```python
from build123d import *

# Parameters (mm, degrees)
F1_DEPTH = 21
F2_R     = 5
F3_R     = 2
F4_DEPTH = 25
F5_R     = 4.5
F6_DEPTH = 4
F7_R     = 3


with BuildPart() as f1:
    # F0 (on Front) → F1 (new body)
    with BuildSketch(Plane.XZ):
        Polygon((95.5, 17), (6.891753, 17), (0, 17), (0, 0), (95.5, 0), align=None)
    extrude(amount=F1_DEPTH)

    # F2
    f2_edges = [f1.edges().sort_by_distance(p)[0] for p in [
        (95.5, -10.5, 17),
    ]]
    fillet(f2_edges, radius=F2_R)

    # F3 (on face) → F4 (cut)
    with BuildSketch(Plane.XY.offset(17)):
        with BuildLine():
            ThreePointArc((41.5, -10.5), (39.5, -8.5), (37.5, -10.5))
            ThreePointArc((37.5, -10.5), (39.5, -12.5), (41.5, -10.5))
        make_face()
        with BuildLine():
            ThreePointArc((7.75, -10.5), (9.75, -12.5), (11.75, -10.5))
            Line((11.75, -10.5), (7.75, -10.5))
        make_face()
        with BuildLine():
            Line((7.75, -10.5), (11.75, -10.5))
            ThreePointArc((11.75, -10.5), (9.75, -8.5), (7.75, -10.5))
        make_face()
        with Locations((78.5, -10.5)):
            Circle(F3_R)
    extrude(amount=-F4_DEPTH, mode=Mode.SUBTRACT)

    # F5 (on face) → F6 (cut)
    with BuildSketch(Plane.XY.offset(17)):
        with Locations((9.75, -10.5)):
            Circle(F5_R)
        with Locations((39.5, -10.5)):
            Circle(F5_R)
        with Locations((78.5, -10.5)):
            Circle(F5_R)
    extrude(amount=-F6_DEPTH, mode=Mode.SUBTRACT)

    # F7
    f7_edges = [f1.edges().sort_by_distance(p)[0] for p in [
        (0, -10.5, 17),
    ]]
    fillet(f7_edges, radius=F7_R)


solid = f1.part
```
Read the model definition and answer for the solid it produces. Units are mm, in the model's axes. A direction names the side the tool comes from. Give positions to 0.01 mm unless a question says otherwise; leave off trailing zeros. Order: outer loops, then holes, each group sorted by start corner. A loop starts at its lowest first (then second) coordinate and runs counter-clockwise, first axis right, second up. Notation, with made-up numbers: (28, -17.75) -> (36, -17.75) arc R31 cw to (36, 20.25) -> close; hole circle Ø9 at (67.5, 34.25). An arc over 180 degrees is marked (long way). One line per item, written item: value. Start each with the question number.
(1) The part is cut by section B-B (x = 9.75). Determine the outline of the cut face in (y, z).
(2) The part is cut by section A-A (z = 7.5). Determine the outline of the cut face in (x, y).
(3) A tool of negligible diameter and unlimited length cuts with its end or side. For faces 1 (the flat face through (10.69, -12.44, 13)), 2 (the flat face through (47, -10, 17)), from which of +Z, -Z, +X, -X, +Y, -Y can it reach the whole face along a straight path? Write none if from no direction.
(4) Straight lines are drawn through the part: L1, parallel to Y at x = 9.75, z = 5; L2, parallel to Y at x = 39.5, z = 16.25; L3, parallel to X at y = -11.75, z = 11.75. For each, find the intervals that lie inside material, in ascending order.
(5) Flat-ended cylindrical pins translate along their axes: P1, Ø2.5, axis at x = 39, y = -9.5, coming from the +Z side; P2, Ø10, axis at x = 12, y = -10, coming from the +Z side; P3, Ø3.5, axis at x = 39.5, y = -10.5, coming from the -Z side; P4, Ø1.5, axis at y = -9, z = 13.5, coming from the +X side. Find the tip coordinate at first contact, or state that the pin passes through.
(6) The part is cut by section C-C (y = -10.5). State how many separate pieces and enclosed holes the cut face has, and give its area (3 significant figures).
(7) For a pull along X with two mould halves and no side action, classify faces 3 (the cylindrical face through (9.49, -8.517, 6.591)), 4 (the flat face through (95.5, -10, 6)), 5 (the flat face through (40.44, -12.44, 13)), 6 (the flat face through (47, 0, 9)) as released by +X, released by -X, zero draft, split by the parting line, or undercut.
Taken from the geometry:
1. outline: (-21, 0) -> (-12.5, 0) -> (-12.5, 13) -> (-15, 13) -> (-15, 17) -> (-21, 17) -> close; (-8.5, 0) -> (0, 0) -> (0, 17) -> (-6, 17) -> (-6, 13) -> (-8.5, 13) -> close
2. outline: (0, -21) -> (95.5, -21) -> (95.5, 0) -> (0, 0) -> close; hole circle Ø4 at (9.75, -10.5); hole circle Ø4 at (39.5, -10.5); hole circle Ø4 at (78.5, -10.5)
3. face 1: +Z
3. face 2: +Z, +X, -X, +Y, -Y
4. L1: -21 to -12.5, -8.5 to 0
4. L2: -21 to -15, -6 to 0
4. L3: 0 to 8.19, 11.31 to 37.94, 41.06 to 76.94, 80.06 to 95.5
5. P1: z = 13
5. P2: z = 17
5. P3: through
5. P4: x = 95.44
6. separate pieces: 4
6. enclosed holes: 0
6. area: 1,350 mm^2
7. face 3: undercut
7. face 4: released by +X
7. face 5: undercut
7. face 6: zero draft
